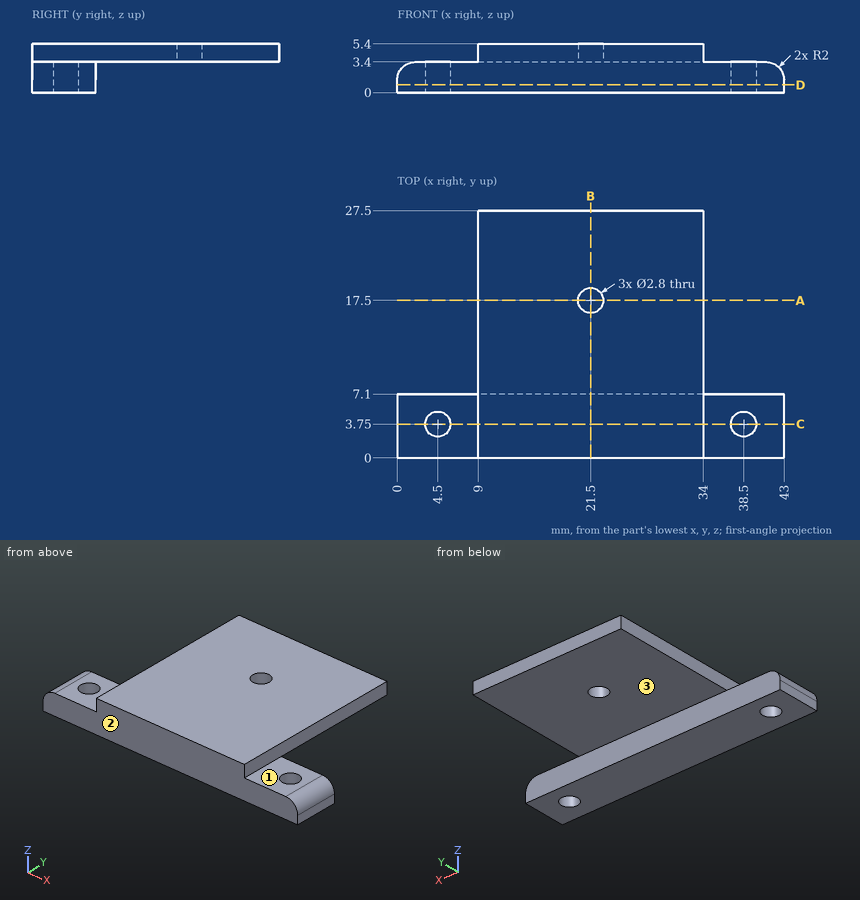
Here's the drawing with two shaded views (mm, measured from the low corner). I have some questions. A direction names the side the tool comes from. Coordinates: 2 decimals unless noted, no trailing zeros. Order: outer loops, then holes, each group sorted by start corner. A loop starts at its lowest first (then second) coordinate and runs counter-clockwise, first axis right, second up. Notation, with made-up numbers: (42, 10) - (52, 10) arc R6 cw to (52, 14) - close; hole circle Ø9 at (-11.5, 13.5). An arc over 180 degrees is marked (long way). Answer in a Markdown table with one row per item. Add a question column.
(1) If we section it at A-A, the plane y = 17.5: Please give me the cut outline in (x, z), then the cut area to 3 significant figures.
(2) I need wall thicknesses on L1, parallel to Y at x = 38.5, z = 1.05; L2, parallel to X at y = 3.75, z = 1.5; L3, parallel to X at y = 17.5, z = 4.9. Which ranges of each line are inside material? Lowest first, please.
(3) On a 3-axis mill with a long thin cutter (end or side, diameter ignored), from which of +Z, -Z, +X, -X, +Y, -Y can I reach the whole of each face in a straight line? I mean the marked faces 1, 2 and 3. Say none if no direction works.
(4) Will these pins go through, and if not, where does the flat tip stop? pin 1 (1.5 mm diameter, centred on y = 6, z = 1, fed in from -X); pin 2 (2 mm diameter, centred on y = 12.5, z = 5, fed in from -X); pin 3 (10 mm diameter, centred on x = 21, y = 18, fed in from -Z); pin 4 (5.5 mm diameter, centred on x = 37, y = 3.5, fed in from +Z).
(5) If we section it at B-B, the plane x = 21.5: Please give me the cut outline in (y, z), then the cut area to 3 significant figures.
(6) If we section it at D-D, the plane z = 0.85: Please give me the cut outline in (x, y).
(7) If we section it at C-C, the plane y = 3.75: Please give me the cut outline in (x, z).
Results are:
| question | item | result |
|---|---|---|
| 1 | outline | (9, 3.4) - (20.1, 3.4) - (20.1, 5.4) - (9, 5.4) - close; (22.9, 3.4) - (34, 3.4) - (34, 5.4) - (22.9, 5.4) - close |
| 1 | area | 44.4 mm2 |
| 2 | L1 | y = 0 to 2.35, 5.15 to 7.1 |
| 2 | L2 | x = 0 to 3.1, 5.9 to 37.1, 39.9 to 43 |
| 2 | L3 | x = 9 to 20.1, 22.9 to 34 |
| 3 | face 1 | +Z, +X, +Y, -Y |
| 3 | face 2 | +Z, -Z, +X, -X, -Y |
| 3 | face 3 | -Z, +X, -X, +Y |
| 4 | pin 1 | stops at x = 0 |
| 4 | pin 2 | stops at x = 9 |
| 4 | pin 3 | stops at z = 3.4 |
| 4 | pin 4 | stops at z = 3.4 |
| 5 | outline | (0, 0) - (7.1, 0) - (7.1, 3.4) - (16.1, 3.4) - (16.1, 5.4) - (0, 5.4) - close; (18.9, 3.4) - (27.5, 3.4) - (27.5, 5.4) - (18.9, 5.4) - close |
| 5 | area | 73.5 mm2 |
| 6 | outline | (0, 0) - (43, 0) - (43, 7.1) - (0, 7.1) - close; hole circle Ø2.8 at (4.5, 3.75); hole circle Ø2.8 at (38.5, 3.75) |
| 7 | outline | (0, 0) - (3.1, 0) - (3.1, 3.4) - (2, 3.4) arc R2 ccw to (0, 1.4) - close; (5.9, 0) - (37.1, 0) - (37.1, 3.4) - (34, 3.4) - (34, 5.4) - (9, 5.4) - (9, 3.4) - (5.9, 3.4) - close; (39.9, 0) - (43, 0) - (43, 1.4) arc R2 ccw to (41, 3.4) - (39.9, 3.4) - close |
